Read the model definition and answer for the solid it produces. Units are mm, in the model's axes. Give positions to 0.01 mm unless a question says otherwise; leave off trailing zeros. Loops run counter-clockwise (first coordinate to the right, second up) from the corner with the lowest first, then second, coordinate; pieces in that order, holes last. Notation, with made-up numbers: (-6.75, 5) - (29.25, 5) arc R12 cw to (29.25, 13) - close; hole circle Ø6 at (12, 65.25). An arc over 180 degrees is marked (long way). Use a Markdown table: item, result. Add a question column.
Item 1: A cutting plane is placed at D-D (x = -12). Determine the outline of the cut face in (y, z), plus the area to 3 significant figures.
Item 2: A cutting plane is placed at C-C (x = 7.5). Determine the outline of the cut face in (y, z).
Item 3: A cutting plane is placed at B-B (z = 34). Determine the outline of the cut face in (x, y), plus the area to 3 significant figures.
Item 4: A cutting plane is placed at A-A (x = 15). Determine the outline of the cut face in (y, z), plus the area to 3 significant figures.
Item 5: Consider probe 1 along X at (y, z) = (1.9, 33.5); probe 2 along Z at (x, y) = (9.5, 0.4); probe 3 along Z at (x, y) = (7, 0.45). Determine where each line is inside the solid, lowest interval first. Write a range as [from, to].
Item 6: This flat-tipped pin is pushed along its axis until it touches: P1, Ø0.6, axis at y = 0.5, z = 34.5, coming from the +X side. Where does it stop, or does it pass through?
from build123d import *

# Parameters (mm, degrees)
IZIM1_R                     = 2
Y_KSEKLIK_EKSTR_ZYON1_DEPTH = 2


with BuildPart() as part:
    # Çizim1 → Yükseklik-Ekstrüzyon1 (new body)
    # profile 1 of 2: a face of its own
    with BuildSketch(Plane(origin=(0, 0, 0), x_dir=(1, 0, 0), z_dir=(0, 1, 0))):
        with BuildLine():
            Line((-2.151853537, -38.922725918), (-2.151853537, -29.922725918))
            ThreePointArc((-2.151853537, -29.922725918), (-29.980675255, 1.076620282), (0, 30))
            Line((0, 30), (0, 35.6))
            ThreePointArc((0, 35.6), (-13.229776272, 33.050461718), (-24.564618776, 25.767023584))
            add(Edge.make_bspline(
                [(-24.564618776, 25.767023584), (-32.251007767, 18.439315954), (-35.719007685, 6.21673721), (-34.276517941, -5.541694008), (-33.608104639, -8.414682353)],
                knots=[0, 0, 0, 0, 0.765438226, 1, 1, 1, 1], degree=3))
            add(Edge.make_bspline(
                [(-33.608104639, -8.414682353), (-31.608167264, -17.010855942), (-25.43277753, -22.569195675), (-19.499413864, -27.49500702)],
                knots=[0, 0, 0, 0, 1, 1, 1, 1], degree=3))
            Line((-19.499413864, -27.49500702), (-17.70199444, -34.827578129))
            ThreePointArc((-17.70199444, -34.827578129), (-10.192020163, -37.881778178), (-2.151853537, -38.922725918))
        make_face()
        with Locations(Location((-6.368896391, -34.390315296, 0), (0, 0, 270))):
            Circle(IZIM1_R, mode=Mode.SUBTRACT)
    # profile 2 of 2: a face of its own
    with BuildSketch(Plane(origin=(0, 0, 0), x_dir=(1, 0, 0), z_dir=(0, 1, 0))):
        with BuildLine():
            ThreePointArc((6.368896391, -29.316158663), (4.271156259, -29.694397185), (2.151853537, -29.922725918))
            Line((2.151853537, -29.922725918), (2.151853537, -38.922725918))
            ThreePointArc((2.151853537, -38.922725918), (10.192020163, -37.881778178), (17.70199444, -34.827578129))
            Line((17.70199444, -34.827578129), (19.499413864, -27.49500702))
            add(Edge.make_bspline(
                [(33.608104639, -8.414682353), (31.608167264, -17.010855942), (25.43277753, -22.569195675), (19.499413864, -27.49500702)],
                knots=[0, 0, 0, 0, 1, 1, 1, 1], degree=3))
            add(Edge.make_bspline(
                [(24.564618776, 25.767023584), (32.251007767, 18.439315954), (35.719007685, 6.21673721), (34.276517941, -5.541694008), (33.608104639, -8.414682353)],
                knots=[0, 0, 0, 0, 0.765438226, 1, 1, 1, 1], degree=3))
            ThreePointArc((24.564618776, 25.767023584), (13.229776272, 33.050461718), (0, 35.6))
            Line((0, 35.6), (0, 30))
            ThreePointArc((0, 30), (21.213203436, 21.213203436), (30, 0))
            ThreePointArc((30, 0), (23.356657421, -18.827282176), (6.368896391, -29.316158663))
        make_face()
        with Locations(Location((6.368896391, -34.390315296, 0), (0, 0, 270))):
            Circle(IZIM1_R, mode=Mode.SUBTRACT)
    extrude(amount=Y_KSEKLIK_EKSTR_ZYON1_DEPTH)


solid = part.part
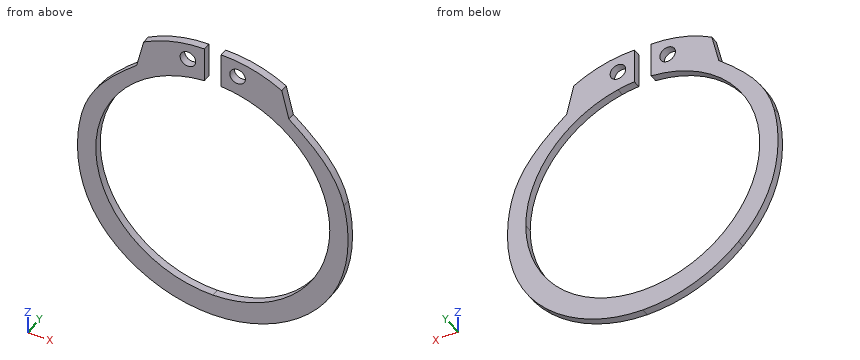
Geometry says:
| question | item | result |
|---|---|---|
| 1 | outline | (0, -33.52) - (2, -33.52) - (2, -27.5) - (0, -27.5) - close; (0, 27.5) - (2, 27.5) - (2, 37.35) - (0, 37.35) - close |
| 1 | area | 31.7 mm² |
| 2 | outline | (0, -34.8) - (2, -34.8) - (2, -29.05) - (0, -29.05) - close; (0, 29.05) - (2, 29.05) - (2, 32.74) - (0, 32.74) - close; (0, 36.04) - (2, 36.04) - (2, 38.47) - (0, 38.47) - close |
| 3 | outline | (-17.9, 0) - (-8.33, 0) - (-8.33, 2) - (-17.9, 2) - close; (-4.41, 0) - (-2.15, 0) - (-2.15, 2) - (-4.41, 2) - close; (2.15, 0) - (4.41, 0) - (4.41, 2) - (2.15, 2) - close; (8.33, 0) - (17.9, 0) - (17.9, 2) - (8.33, 2) - close |
| 3 | area | 47.3 mm² |
| 4 | outline | (0, -32.29) - (2, -32.29) - (2, -25.98) - (0, -25.98) - close; (0, 25.98) - (2, 25.98) - (2, 36.19) - (0, 36.19) - close |
| 4 | area | 33.0 mm² |
| 5 | probe 1 | [-18.03, -8.16], [-4.58, -2.15], [2.15, 4.58], [8.16, 18.03] |
| 5 | probe 2 | [-34.31, -28.46], [28.46, 38.06] |
| 5 | probe 3 | [-34.91, -29.17], [29.17, 32.49], [36.29, 38.55] |
| 6 | P1 | x = 17.86 |
